Design review of the part built by this model. Coordinates are the model's own, in mm. Give positions to 0.01 mm unless a question says otherwise; leave off trailing zeros. Order: outer loops, then holes, each group sorted by start corner. A loop starts at its lowest first (then second) coordinate and runs counter-clockwise, first axis right, second up. Notation, with made-up numbers: (-0.5, 81) -> (39.5, 81) arc R6 cw to (39.5, 89) -> close; hole circle Ø4 at (75.5, 72). An arc over 180 degrees is marked (long way). Answer in a Markdown table with one row per item. Add a question column.
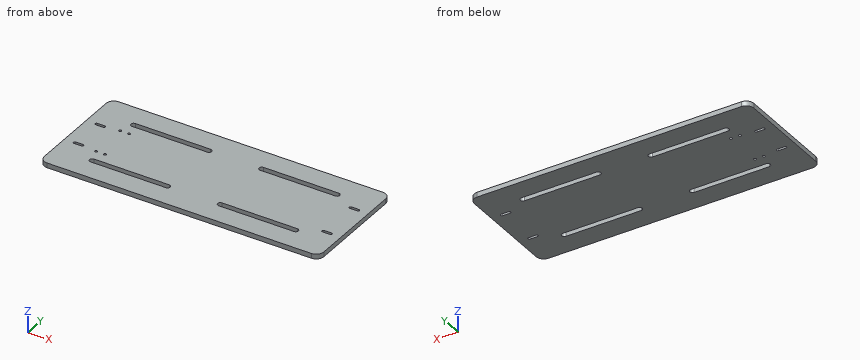
```python
from build123d import *

# Parameters (mm, degrees)
SKETCH1_W           = 370.84
SKETCH1_H           = 150
BOSS_EXTRUDE1_DEPTH = 6.35
FILLET3_R           = 10
FILLET4_R           = 10
FILLET5_R           = 10
FILLET6_R           = 10
SKETCH3_R           = 1.7
CUT_EXTRUDE1_DEPTH  = 10
CUT_EXTRUDE2_DEPTH  = 10
SKETCH6_R           = 1.7
CUT_EXTRUDE3_DEPTH  = 7.35


with BuildPart() as part:
    # Sketch1 → Boss-Extrude1 (new body)
    with BuildSketch(Plane.XY):
        with Locations((185.42, -75)):
            Rectangle(SKETCH1_W, SKETCH1_H)
    extrude(amount=BOSS_EXTRUDE1_DEPTH)

    # Fillet3
    fillet3_edges = [part.edges().sort_by_distance(p)[0] for p in [
        (0, 0, 3.175),
    ]]
    fillet(fillet3_edges, radius=FILLET3_R)

    # Fillet4
    fillet4_edges = [part.edges().sort_by_distance(p)[0] for p in [
        (0, -150, 3.175),
    ]]
    fillet(fillet4_edges, radius=FILLET4_R)

    # Fillet5
    fillet5_edges = [part.edges().sort_by_distance(p)[0] for p in [
        (370.84, -150, 3.175),
    ]]
    fillet(fillet5_edges, radius=FILLET5_R)

    # Fillet6
    fillet6_edges = [part.edges().sort_by_distance(p)[0] for p in [
        (370.84, 0, 3.175),
    ]]
    fillet(fillet6_edges, radius=FILLET6_R)

    # Sketch3 → Cut-Extrude1 (cut)
    with BuildSketch(Plane.XY.offset(6.35)):
        with Locations((18.62, -52.205)):
            Circle(SKETCH3_R)
        with Locations((18.62, -97.795)):
            Circle(SKETCH3_R)
        with Locations((352.22, -103.75)):
            Circle(SKETCH3_R)
        with Locations((352.22, -46.25)):
            Circle(SKETCH3_R)
    extrude(amount=-CUT_EXTRUDE1_DEPTH, mode=Mode.SUBTRACT)

    # Sketch4 → Cut-Extrude2 (cut)
    with BuildSketch(Plane.XY.offset(6.35)):
        with BuildLine():
            Line((50, -28), (150, -28))
            ThreePointArc((150, -28), (153.5, -31.5), (150, -35))
            Line((150, -35), (50, -35))
            ThreePointArc((50, -35), (46.5, -31.5), (50, -28))
        make_face()
        with BuildLine():
            Line((220, -28), (320, -28))
            ThreePointArc((320, -28), (323.5, -31.5), (320, -35))
            Line((320, -35), (220, -35))
            ThreePointArc((220, -35), (216.5, -31.5), (220, -28))
        make_face()
        with BuildLine():
            Line((50, -115), (150, -115))
            ThreePointArc((150, -115), (153.5, -118.5), (150, -122))
            Line((150, -122), (50, -122))
            ThreePointArc((50, -122), (46.5, -118.5), (50, -115))
        make_face()
        with BuildLine():
            Line((220, -115), (320, -115))
            ThreePointArc((320, -115), (323.5, -118.5), (320, -122))
            Line((320, -122), (220, -122))
            ThreePointArc((220, -122), (216.5, -118.5), (220, -115))
        make_face()
    extrude(amount=-CUT_EXTRUDE2_DEPTH, mode=Mode.SUBTRACT)

    # Sketch6 → Cut-Extrude3 (cut, through all)
    with BuildSketch(Plane.XY.offset(6.35)):
        with Locations((43.62, -49.75)):
            Circle(SKETCH6_R)
        with Locations((43.62, -100.25)):
            Circle(SKETCH6_R)
        with Locations((55.42, -49.75)):
            Circle(SKETCH6_R)
        with Locations((55.42, -100.25)):
            Circle(SKETCH6_R)
        with BuildLine():
            Line((13.62, -50.505), (23.62, -50.505))
            ThreePointArc((23.62, -50.505), (25.32, -52.205), (23.62, -53.905))
            Line((23.62, -53.905), (13.62, -53.905))
            ThreePointArc((13.62, -53.905), (11.92, -52.205), (13.62, -50.505))
        make_face()
        with BuildLine():
            Line((13.62, -96.095), (23.62, -96.095))
            ThreePointArc((23.62, -96.095), (25.32, -97.795), (23.62, -99.495))
            Line((23.62, -99.495), (13.62, -99.495))
            ThreePointArc((13.62, -99.495), (11.92, -97.795), (13.62, -96.095))
        make_face()
        with BuildLine():
            Line((347.22, -44.525), (357.22, -44.525))
            ThreePointArc((357.22, -44.525), (358.945, -46.25), (357.22, -47.975))
            Line((357.22, -47.975), (347.22, -47.975))
            ThreePointArc((347.22, -47.975), (345.495, -46.25), (347.22, -44.525))
        make_face()
        with BuildLine():
            Line((347.22, -102.025), (357.22, -102.025))
            ThreePointArc((357.22, -102.025), (358.945, -103.75), (357.22, -105.475))
            Line((357.22, -105.475), (347.22, -105.475))
            ThreePointArc((347.22, -105.475), (345.495, -103.75), (347.22, -102.025))
        make_face()
    extrude(amount=-CUT_EXTRUDE3_DEPTH, mode=Mode.SUBTRACT)


solid = part.part
```
1) Clearance check with a flat-ended pin moving along its axis: P1, Ø3, axis at x = 43.62, y = -100.25, coming from the -Z side. State where the tip first meets the part, or that it passes through.
2) For L1, parallel to Y at x = 287, z = 2; L2, parallel to X at y = -100.25, z = 3.5; L3, parallel to X at y = -28.5, z = 2, list the stretches that pass through material, from the lowest coordinate up.
3) Add section A-A, the plane x = 300.5. Write out the cut boundary in (y, z).
4) Add section B-B, the plane z = 4. Give the number of separate pieces and of enclosed holes in the cut face, and give its area (3 significant figures).
Verdict:
| question | item | result |
|---|---|---|
| 1 | P1 | passes through |
| 2 | L1 | y = -150 to -122, -115 to -35, -28 to 0 |
| 2 | L2 | x = 0 to 41.92, 45.32 to 53.72, 57.12 to 370.84 |
| 2 | L3 | x = 0 to 48.2, 151.8 to 218.2, 321.8 to 370.84 |
| 3 | outline | (-150, 0) -> (-122, 0) -> (-122, 6.35) -> (-150, 6.35) -> close; (-115, 0) -> (-35, 0) -> (-35, 6.35) -> (-115, 6.35) -> close; (-28, 0) -> (0, 0) -> (0, 6.35) -> (-28, 6.35) -> close |
| 4 | separate pieces | 1 |
| 4 | enclosed holes | 12 |
| 4 | area | 52,400 mm2 |
